from build123d import *

# Parameters (mm, degrees)
FILLET2_R  = 0.9
SKETCH2_W  = 5.6
SKETCH2_H  = 0.8
SLOT_DEPTH = 0.7


with BuildPart() as part:
    # BodySke → Base-Revolve (revolve)
    with BuildSketch(Plane.XY, mode=Mode.PRIVATE) as base_revolve_sk:
        Polygon((1.8, 1.5), (1.8, 2.8), (0, 2.642520406), (0, 0), (26.8, 0), (26.8, 1.5), align=None)
    revolve(base_revolve_sk.sketch.rotate(Axis((-25.4, 0, 0), (1, 0, 0)), 90), axis=Axis((-25.4, 0, 0), (1, 0, 0)))

    # Fillet2
    fillet2_edges = [part.edges().sort_by_distance(p)[0] for p in [
        (0, 0, -2.642520406),
    ]]
    fillet(fillet2_edges, radius=FILLET2_R)

    # Sketch2 → Slot (cut)
    with BuildSketch(Plane(origin=(0, 0, 0), x_dir=(0, 0, -1), z_dir=(1, 0, 0))):
        Rectangle(SKETCH2_W, SKETCH2_H)
    extrude(amount=SLOT_DEPTH, mode=Mode.SUBTRACT)

    # ThdSchSke → ThreadSchematic (revolve, cut)
    with BuildSketch(Plane.XY):
        Polygon((2.8, -1.2195), (2.603591786, -1.5), (2.603591786, -1.875), (2.996408214, -1.875), (2.996408214, -1.5), align=None)
    revolve(axis=Axis((-3.175, 0, 0), (1, 0, 0)), mode=Mode.SUBTRACT)


solid = part.part
Build history of the part. All positions in model axes, mm. A direction names the side the tool comes from. Round coordinates to 2 decimals unless told otherwise and drop trailing zeros. Write each loop counter-clockwise with the first axis right and the second up, starting at its lowest first coordinate (ties: lowest second). Pieces come first, ordered by that corner, then holes. Notation, with made-up numbers: M 56,74.25 L 79,74.25 A15 ccw 79,85.25 Z; hole C 14.25,63 d7. An arc over 180 degrees is marked long. Answer as a JSON object with one key per item and string values. Group by question number.
(1) Cut at B-B (y = 0). Give the cut face in (x, z), and give its area (3 significant figures).
(2) Cut at A-A (z = 0). Give the cut face in (x, y), and give its area (3 significant figures).
(3) Mould opens along X. For faces 4 (the cylindrical face through (14.73, -0.45, 1.43)), 5 (the flat face through (26.8, 0, 0)), 6 (the flat face through (0, -1, 0)) say: pulls with the +X half, pulls with the -X half, needs draft (parallel to the pull), parting line crosses it, or undercut.
(4) Drill centre lines: L1, parallel to Z at x = 19.25, y = 0.1; L2, parallel to X at y = 0.05, z = 2; L3, parallel to X at y = -0.3, z = 1.4. Where is each one in solid material? Low to high.
(5) Flat gauge pins, fed straight in: pin 1 (1.5 mm diameter, centred on x = 20, z = 1, fed in from -Y); pin 2 (0.6 mm diameter, centred on x = 0.5, z = -1, fed in from -Y). Where does each tip first touch, or does it go through?
(6) Which spindle directions (+Z, -Z, +X, -X, +Y, -Y) get a long thin tool onto all of the face, cutting with end or side? Do faces 1 (the flat face through (0.7, 0, 0)), 2 (the flat face through (0, 1, 0)), 3 (the flat face through (1.8, 1.2, -1.2)). Say none if no direction does.
(7) Cut at C-C (x = 9). Give the cut face in (y, z), and give its area (3 significant figures).
Responses:
{
 "1": {"outline": "M 0.7,-2.7 A0.9 ccw 0.82,-2.71 L 1.8,-2.8 L 1.8,-1.5 L 2.6,-1.5 L 2.8,-1.22 L 3,-1.5 L 26.8,-1.5 L 26.8,1.5 L 3,1.5 L 2.8,1.22 L 2.6,1.5 L 1.8,1.5 L 1.8,2.8 L 0.82,2.71 A0.9 ccw 0.7,2.7 Z", "area": "80.9 mm2"},
 "2": {"outline": "M 0,-1.82 A0.9 ccw 0.82,-2.71 L 1.8,-2.8 L 1.8,-1.5 L 2.6,-1.5 L 2.8,-1.22 L 3,-1.5 L 26.8,-1.5 L 26.8,1.5 L 3,1.5 L 2.8,1.22 L 2.6,1.5 L 1.8,1.5 L 1.8,2.8 L 0.82,2.71 A0.9 ccw 0,1.82 L 0,0.4 L 0.7,0.4 L 0.7,-0.4 L 0,-0.4 Z", "area": "83.8 mm2"},
 "3": {"face 4": "needs draft", "face 5": "pulls with the +X half", "face 6": "pulls with the -X half"},
 "4": {"L1": "z = -1.5 to 1.5", "L2": "x = 0.7 to 1.8", "L3": "x = 0.7 to 2.65, 2.95 to 26.8"},
 "5": {"pin 1": "stops at y = -1.48", "pin 2": "stops at y = -2.58"},
 "6": {"face 1": "+Z, -Z, -X", "face 2": "+Z, -Z, -X, +Y, -Y", "face 3": "+X"},
 "7": {"outline": "C 0,0 d3", "area": "7.07 mm2"}
}
